from build123d import *

# Parameters (mm, degrees)
BOSS_EXTRUDE1_DEPTH = 12
SKETCH2_R           = 1.7
BOSS_EXTRUDE2_DEPTH = 6.2125


with BuildPart() as part:
    # Sketch1 → Boss-Extrude1 (new body)
    with BuildSketch(Plane(origin=(0, 0, 0), x_dir=(1, 0, 0), z_dir=(0, 1, 0))):
        Polygon((10.15, -65.254427144), (6.15, -65.254427144), (6.15, -66.934427144), (-6.15, -66.934427144), (-6.15, -65.254427144), (-10.15, -65.254427144), (-10.15, -56.819346079), (10.15, -56.819346079), align=None)
    extrude(amount=BOSS_EXTRUDE1_DEPTH)

    # Sketch2 → Boss-Extrude2 (add, symmetric)
    with BuildSketch(Plane(origin=(0, 0, 0), x_dir=(0, 0, -1), z_dir=(1, 0, 0))):
        with BuildLine():
            Line((-72.207292933, 5.999665069), (-72.207292933, 8.809665069))
            ThreePointArc((-72.207292933, 8.809665069), (-70.065734946, 11.180872507), (-66.977292933, 11.999665069))
            Line((-66.977292933, 11.999665069), (-66.934427144, 12))
            Line((-66.934427144, 12), (-66.934427144, 0))
            Line((-66.934427144, 0), (-72.207292933, 0))
            Line((-72.207292933, 0), (-72.207292933, 5.999665069))
        make_face()
        with Locations((-69.217292933, 8.579665069)):
            Circle(SKETCH2_R, mode=Mode.SUBTRACT)
    extrude(amount=BOSS_EXTRUDE2_DEPTH, both=True)


solid = part.part
Work out the finished part from the listing and answer in its coordinate system (mm). A direction names the side the tool comes from. Coordinates: 2 decimals unless noted, no trailing zeros. Loops run counter-clockwise (first coordinate to the right, second up) from the corner with the lowest first, then second, coordinate; pieces in that order, holes last. Notation, with made-up numbers: M -21,27 L 26,27 A30 ccw 26,62 Z; hole C 84,-26 d6. An arc over 180 degrees is marked long. Answer in a Markdown table with one row per item. Add a question column.
1. Find section B-B, the plane x = -0.5. Write down the section's boundary in (y, z).
2. The mould has two halves that part along Z. Classify faces 4 (the flat face through (6.15, 6, 66)), 5 (the cylindrical face through (-0.087, 8.654, 70.916)), 6 (the flat face through (6.212, 5, 70)), 7 (the flat face through (0, 6, 56.819)): pulls with the +Z half, pulls with the -Z half, needs draft (parallel to the pull), parting line crosses it, or undercut.
3. Find section C-C, the plane y = 7.75. Write down the section's boundary in (x, z).
4. Find section A-A, the plane z = 70.5. Write down the section's boundary in (x, y).
5. Find section D-D, the plane z = 68. Write down the section's boundary in (x, y).
6. Consider L1, parallel to Z at x = -7.5, y = 9; L2, parallel to Y at x = 0.5, z = 61; L3, parallel to Y at x = -0.25, z = 68.5. Determine where each line is inside the solid, lowest interval first.
7. A tool of negligible diameter and unlimited length cuts with its end or side. For faces 1 (the flat face through (-6.212, 5, 70)), 2 (the flat face through (-10.15, 6, 61)), 3 (the flat face through (-6.15, 6, 66)), from which of +Z, -Z, +X, -X, +Y, -Y can it reach the whole face along a straight path? Write none if from no direction.
8. Flat-ended cylindrical pins translate along their axes: P1, Ø4, axis at y = 7.5, z = 69, coming from the +X side; P2, Ø3, axis at x = 7, z = 69, coming from the +Y side; P3, Ø2, axis at x = -8.5, y = 3, coming from the +Z side. Find the tip coordinate at first contact, or state that the pin passes through.
Reported:
| question | item | result |
|---|---|---|
| 1 | outline | M 0,56.82 L 12,56.82 L 12,66.93 L 12,66.98 A5.61 ccw 8.81,72.21 L 0,72.21 Z; hole C 8.58,69.22 d3.4 |
| 2 | face 4 | undercut |
| 2 | face 5 | undercut |
| 2 | face 6 | needs draft |
| 2 | face 7 | pulls with the -Z half |
| 3 | outline | M -10.15,56.82 L 10.15,56.82 L 10.15,65.25 L 6.15,65.25 L 6.15,66.93 L 6.21,66.93 L 6.21,67.73 L -6.21,67.73 L -6.21,66.93 L -6.15,66.93 L -6.15,65.25 L -10.15,65.25 Z; M -6.21,70.7 L 6.21,70.7 L 6.21,72.21 L -6.21,72.21 Z |
| 4 | outline | M -6.21,0 L 6.21,0 L 6.21,7.46 L -6.21,7.46 Z; M -6.21,9.7 L 6.21,9.7 L 6.21,10.89 L -6.21,10.89 Z |
| 5 | outline | M -6.21,0 L 6.21,0 L 6.21,7.39 L -6.21,7.39 Z; M -6.21,9.77 L 6.21,9.77 L 6.21,11.94 L -6.21,11.94 Z |
| 6 | L1 | z = 56.82 to 65.25 |
| 6 | L2 | y = 0 to 12 |
| 6 | L3 | y = 0 to 7.04, 10.12 to 11.84 |
| 7 | face 1 | +Z, -X, +Y, -Y |
| 7 | face 2 | +Z, -Z, -X, +Y, -Y |
| 7 | face 3 | -X, +Y, -Y |
| 8 | P1 | stops at x = 6.21 |
| 8 | P2 | stops at y = 11.97 |
| 8 | P3 | stops at z = 65.25 |
